Design review of the part shown in the three views and the two pictorial views. Dimensions are in mm from the part's minimum x, y and z. A direction names the side the tool comes from. Round coordinates to 2 decimals unless told otherwise and drop trailing zeros. Loops run counter-clockwise (first coordinate to the right, second up) from the corner with the lowest first, then second, coordinate; pieces in that order, holes last.
1. To check wall thickness, follow line 1 along Y through (x, z) = (29.25, 20); line 2 along X through (y, z) = (31, 46.5); line 3 along Z through (x, y) = (32.5, 32). State the ranges of each line that lie inside material, in increasing order.
2. Consider section C-C on x = 30. State the section outline as (y, z) points, then the cut area to 3 significant figures.
3. Tool access review of the marked faces 1, 2 and 3: name each direction out of +Z, -Z, +X, -X, +Y, -Y from which nothing blocks a thin tool from reaching the whole face with its end or side.
4. Clearance check with flat-ended pins moving along their axes: pin 1 Ø15 at (y, z) = (30, 20) entering from +X; pin 2 Ø3 at (x, y) = (13, 10.5) entering from -Z; pin 3 Ø4 at (y, z) = (39, 64.5) entering from +X; pin 4 Ø10 at (y, z) = (37, 26) entering from -X. State where each tip first meets the part, or that it passes through.
5. Consider section A-A on z = 20. State the section outline as (x, y) points, then the cut area to 3 significant figures.
6. Consider section B-B on y = 30. State the section outline as (x, z) points, then the cut area to 3 significant figures.
7. Draft analysis for pull direction Y (two halves, no side actions). For the marked faces 4, 5, 6 and 7, state which applies: released by +Y, released by -Y, zero draft, split by the parting line, or undercut.
8. Consider section D-D on x = 47. State the section outline as (y, z) points.
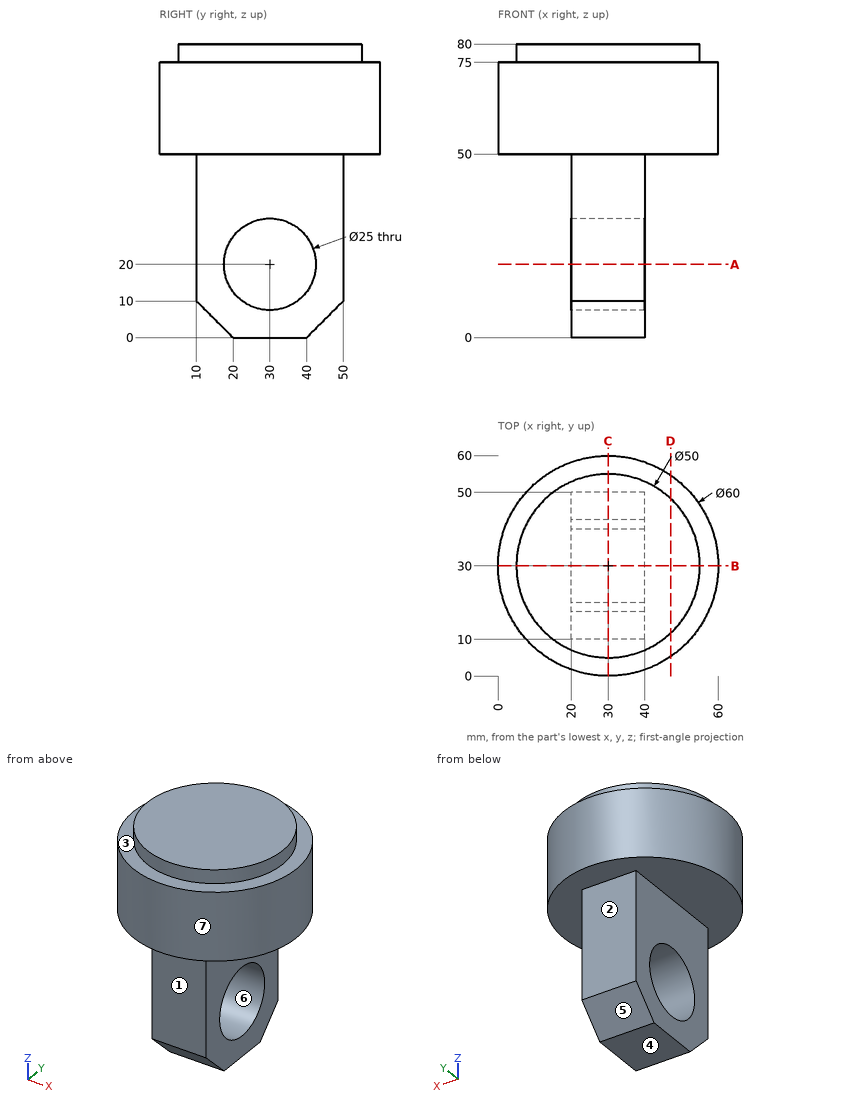
Resolved:
1. line 1: y = 10 to 17.5, 42.5 to 50
1. line 2: x = 20 to 40
1. line 3: z = 0 to 7.66, 32.34 to 80
2. outline: (0, 50) - (10, 50) - (10, 10) - (20, 0) - (40, 0) - (50, 10) - (50, 50) - (60, 50) - (60, 75) - (55, 75) - (55, 80) - (5, 80) - (5, 75) - (0, 75) - close; hole circle Ø25 at (30, 20)
2. area: 3,160 mm2
3. face 1: -Z, +X, -X, -Y
3. face 2: -Z, +X, -X, +Y
3. face 3: +Z
4. pin 1: passes through
4. pin 2: stops at z = 50
4. pin 3: stops at x = 59.17
4. pin 4: stops at x = 20
5. outline: (20, 10) - (40, 10) - (40, 17.5) - (20, 17.5) - close; (20, 42.5) - (40, 42.5) - (40, 50) - (20, 50) - close
5. area: 300 mm2
6. outline: (0, 50) - (20, 50) - (20, 32.5) - (40, 32.5) - (40, 50) - (60, 50) - (60, 75) - (55, 75) - (55, 80) - (5, 80) - (5, 75) - (0, 75) - close; (20, 0) - (40, 0) - (40, 7.5) - (20, 7.5) - close
6. area: 2,250 mm2
7. face 4: zero draft
7. face 5: released by +Y
7. face 6: undercut
7. face 7: split by the parting line
8. outline: (5.28, 50) - (54.72, 50) - (54.72, 75) - (48.33, 75) - (48.33, 80) - (11.67, 80) - (11.67, 75) - (5.28, 75) - close
